Part print with two shaded views. Sizes in mm from the minimum x, y, z corner. Give positions to 0.01 mm unless a question says otherwise; leave off trailing zeros. Order: outer loops, then holes, each group sorted by start corner. A loop starts at its lowest first (then second) coordinate and runs counter-clockwise, first axis right, second up. Notation, with made-up numbers: M 52,72 L 109,72 A20 ccw 109,88 Z; hole C 65.25,26.5 d9. An arc over 180 degrees is marked long. Answer as CSV lines item,"result".
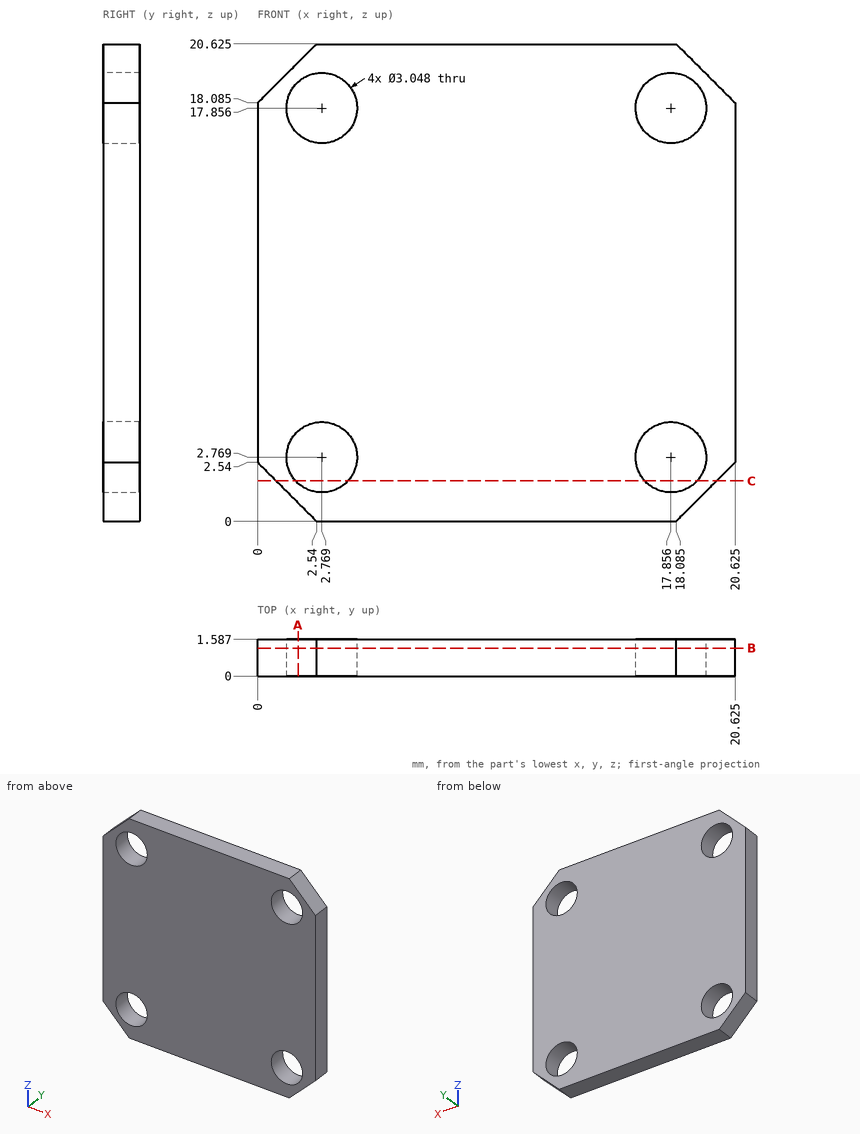
Item 1: Band-saw the part on A-A (x = 1.75). Give the cut face in (y, z) (1 decimal).
Geometry says:
outline,"M 0,0.8 L 1.6,0.8 L 1.6,1.6 L 0,1.6 Z; M 0,3.9 L 1.6,3.9 L 1.6,16.7 L 0,16.7 Z; M 0,19 L 1.6,19 L 1.6,19.8 L 0,19.8 Z"
Item 2: Band-saw the part on B-B (y = 1.2). Give the cut face in (x, z) (1 decimal).
Geometry says:
outline,"M 0,2.5 L 2.5,0 L 18.1,0 L 20.6,2.5 L 20.6,18.1 L 18.1,20.6 L 2.5,20.6 L 0,18.1 Z; hole C 2.8,2.8 d3; hole C 2.8,17.9 d3; hole C 17.9,2.8 d3; hole C 17.9,17.9 d3"
Item 3: Band-saw the part on C-C (z = 1.75). Give the cut face in (x, y) (1 decimal).
Geometry says:
outline,"M 0.8,0 L 1.6,0 L 1.6,1.6 L 0.8,1.6 Z; M 3.9,0 L 16.7,0 L 16.7,1.6 L 3.9,1.6 Z; M 19,0 L 19.8,0 L 19.8,1.6 L 19,1.6 Z"
Item 4: Probe line 1 along X through (y, z) = (1.4, 2.5) (1 decimal); line 2 along Z through (x, y) = (3.25, 0.6) (1 decimal); line 3 along Z through (x, y) = (4, 1.3) (1 decimal). List the from-to ranges inside material, lowest first. Write a range as from..to.
Geometry says:
line 1,"x = 0..1.3, 4.3..16.4, 19.4..20.6"
line 2,"z = 0..1.3, 4.2..16.4, 19.3..20.6"
line 3,"z = 0..1.9, 3.7..17, 18.8..20.6"
